from build123d import *

# Parameters (mm, degrees)
CROQUIS1_W              = 45
CROQUIS1_H              = 15
CROQUIS1_R              = 2.2
SALIENTE_EXTRUIR1_DEPTH = 4
REDONDEO1_R             = 5


with BuildPart() as part:
    # Croquis1 → Saliente-Extruir1 (new body)
    with BuildSketch(Plane.XY):
        with Locations((22.5, 7.5)):
            Rectangle(CROQUIS1_W, CROQUIS1_H)
        with Locations((5, 7.5)):
            Circle(CROQUIS1_R, mode=Mode.SUBTRACT)
        with Locations((40, 7.5)):
            Circle(CROQUIS1_R, mode=Mode.SUBTRACT)
    extrude(amount=SALIENTE_EXTRUIR1_DEPTH)

    # Redondeo1
    redondeo1_edges = [part.edges().sort_by_distance(p)[0] for p in [
        (0, 0, 2),
        (0, 15, 2),
        (45, 15, 2),
        (45, 0, 2),
    ]]
    fillet(redondeo1_edges, radius=REDONDEO1_R)


solid = part.part
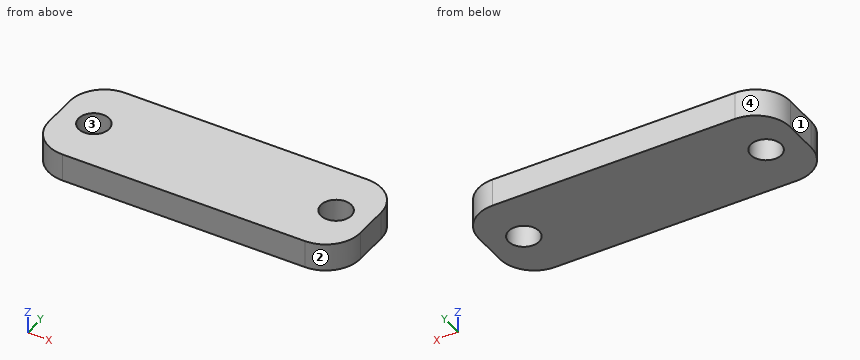
Could you check a few things on this model? Use its own coordinates, in mm. Face numbers are marked on the shaded views. Round coordinates to 2 decimals unless told otherwise and drop trailing zeros. Loops run counter-clockwise (first coordinate to the right, second up) from the corner with the lowest first, then second, coordinate; pieces in that order, holes last. Notation, with made-up numbers: (-22, 83) - (-17, 83) arc R15 cw to (-17, 100) - close; hole circle Ø2 at (-34, 53). An arc over 180 degrees is marked (long way). Write item = value, one per line.
1) If we mould it in two halves opening along Y, with no side actions, what happens to the marked faces 1, 2, 3 and 4? For each: pulls with the +Y half, pulls with the -Y half, needs draft (parallel to the pull), parting line crosses it, or undercut.
Computed:
face_1 = needs draft
face_2 = pulls with the -Y half
face_3 = undercut
face_4 = pulls with the +Y half
2) Imagine slicing it at B-B (z = 0.8). Please give me the cut outline in (x, y), and give its area (3 significant figures).
Computed:
outline = (0, 5) arc R5 ccw to (5, 0) - (40, 0) arc R5 ccw to (45, 5) - (45, 10) arc R5 ccw to (40, 15) - (5, 15) arc R5 ccw to (0, 10) - close; hole circle Ø4.4 at (5, 7.5); hole circle Ø4.4 at (40, 7.5)
area = 623 mm2
3) I need wall thicknesses on line 1 along Y through (x, z) = (5, 1.65); line 2 along Y through (x, z) = (38, 1.9); line 3 along X through (y, z) = (5.75, 2.3). Which ranges of each line are inside material? Lowest first, please. Write a range as from..to.
Computed:
line_1 = 0..5.3, 9.7..15
line_2 = 0..6.58, 8.42..15
line_3 = 0..3.67, 6.33..38.67, 41.33..45
4) Imagine slicing it at A-A (y = 7.5). Please give me the cut outline in (x, z), and give its area (3 significant figures).
Computed:
outline = (0, 0) - (2.8, 0) - (2.8, 4) - (0, 4) - close; (7.2, 0) - (37.8, 0) - (37.8, 4) - (7.2, 4) - close; (42.2, 0) - (45, 0) - (45, 4) - (42.2, 4) - close
area = 145 mm2
5) Imagine slicing it at C-C (y = 12.25). Please give me the cut outline in (x, z).
Computed:
outline = (0.53, 0) - (44.47, 0) - (44.47, 4) - (0.53, 4) - close
6) I'm going to push flat-ended pins straight in: P1, Ø5, axis at x = 40, y = 7.5, coming from the +Z side; P2, Ø1, axis at y = 11, z = 3, coming from the -X side. Where does each tip first touch, or does it pass through?
Computed:
P1 = 4
P2 = 0.03
